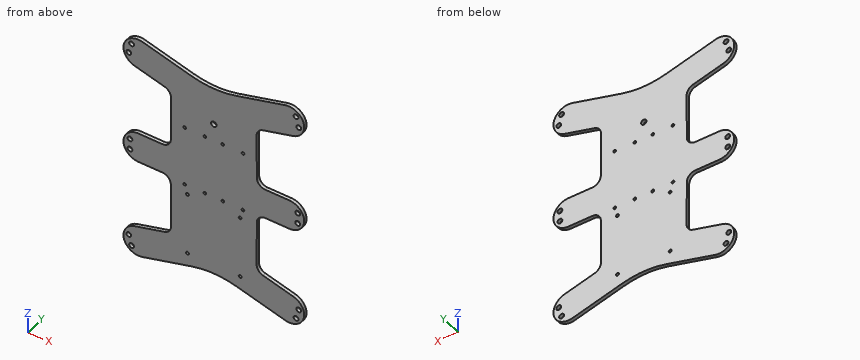
```python
from build123d import *

# Parameters (mm, degrees)
BOSS_EXTRUDE1_DEPTH = 3.175
FILLET1_R           = 80
FILLET2_R           = 8
SKETCH2_R           = 1.35
CUT_EXTRUDE1_DEPTH  = 136.741386774
SKETCH3_R           = 1.25
CUT_EXTRUDE2_DEPTH  = 136.741386774
SKETCH5_R           = 2.55
CUT_EXTRUDE3_DEPTH  = 136.741386774
SKETCH7_R           = 2.25
CUT_EXTRUDE4_DEPTH  = 10


with BuildPart() as part:
    # Sketch1 → Boss-Extrude1 (new body)
    with BuildSketch(Plane(origin=(0, 0, 0), x_dir=(1, 0, 0), z_dir=(0, 1, 0))):
        with BuildLine():
            Line((-70, 14), (-40, 14))
            Line((-40, 14), (-39.816062711, 70))
            Line((-39.816062711, 70), (-73.623466631, 79.058666579))
            ThreePointArc((-73.623466631, 79.058666579), (-83.522961568, 96.205094778), (-66.376533369, 106.104589715))
            Line((-66.376533369, 106.104589715), (0, 88.319051202))
            Line((0, 88.319051202), (66.376533369, 106.104589715))
            ThreePointArc((66.376533369, 106.104589715), (83.522961568, 96.205094778), (73.623466631, 79.058666579))
            Line((73.623466631, 79.058666579), (39.816062711, 70))
            Line((39.816062711, 70), (40, 14))
            Line((40, 14), (70, 14))
            ThreePointArc((70, 14), (84, 0), (70, -14))
            Line((70, -14), (40, -14))
            Line((40, -14), (39.816062711, -70))
            Line((39.816062711, -70), (73.623466631, -79.058666579))
            ThreePointArc((73.623466631, -79.058666579), (83.522961568, -96.205094778), (66.376533369, -106.104589715))
            Line((66.376533369, -106.104589715), (0, -88.319051202))
            Line((0, -88.319051202), (-66.376533369, -106.104589715))
            ThreePointArc((-66.376533369, -106.104589715), (-83.522961568, -96.205094778), (-73.623466631, -79.058666579))
            Line((-73.623466631, -79.058666579), (-39.816062711, -70))
            Line((-39.816062711, -70), (-40, -14))
            Line((-40, -14), (-70, -14))
            ThreePointArc((-70, -14), (-84, 0), (-70, 14))
        make_face()
    extrude(amount=BOSS_EXTRUDE1_DEPTH)

    # Fillet1
    fillet1_edges = [part.edges().sort_by_distance(p)[0] for p in [
        (0, 1.5875, -88.319051202),
        (0, 1.5875, 88.319051202),
    ]]
    fillet(fillet1_edges, radius=FILLET1_R)

    # Fillet2
    fillet2_edges = [part.edges().sort_by_distance(p)[0] for p in [
        (-40, 1.5875, -14),
        (-39.816062711, 1.5875, -70),
        (39.816062711, 1.5875, -70),
        (40, 1.5875, -14),
        (40, 1.5875, 14),
        (39.816062711, 1.5875, 70),
        (-39.816062711, 1.5875, 70),
        (-40, 1.5875, 14),
    ]]
    fillet(fillet2_edges, radius=FILLET2_R)

    # Sketch2 → Cut-Extrude1 (cut, through all)
    with BuildSketch(Plane(origin=(0, 3.175, 0), x_dir=(1, 0, 0), z_dir=(0, 1, 0))):
        with Locations(Location((-24.5, 24.641145635, 0), (0, 0, 270))):
            Circle(SKETCH2_R)
        with Locations(Location((24.5, 24.641145635, 0), (0, 0, 270))):
            Circle(SKETCH2_R)
        with Locations(Location((24.5, 82.641145635, 0), (0, 0, 270))):
            Circle(SKETCH2_R)
        with Locations(Location((-24.5, 82.641145635, 0), (0, 0, 270))):
            Circle(SKETCH2_R)
    extrude(amount=-CUT_EXTRUDE1_DEPTH, mode=Mode.SUBTRACT)

    # Sketch3 → Cut-Extrude2 (cut, through all)
    with BuildSketch(Plane(origin=(0, 3.175, 0), x_dir=(1, 0, 0), z_dir=(0, 1, 0))):
        with Locations(Location((-8.3, -40.058854365, 0), (0, 0, 270))):
            Circle(SKETCH3_R)
        with Locations(Location((-27.1, -40.058854365, 0), (0, 0, 270))):
            Circle(SKETCH3_R)
        with Locations(Location((-27.1, 15.841145635, 0), (0, 0, 270))):
            Circle(SKETCH3_R)
        with Locations(Location((-8.3, 15.841145635, 0), (0, 0, 270))):
            Circle(SKETCH3_R)
        with Locations(Location((8.3, 15.841145635, 0), (0, 0, 270))):
            Circle(SKETCH3_R)
        with Locations(Location((27.1, 15.841145635, 0), (0, 0, 270))):
            Circle(SKETCH3_R)
        with Locations(Location((8.3, -40.058854365, 0), (0, 0, 270))):
            Circle(SKETCH3_R)
        with Locations(Location((27.1, -40.058854365, 0), (0, 0, 270))):
            Circle(SKETCH3_R)
    extrude(amount=-CUT_EXTRUDE2_DEPTH, mode=Mode.SUBTRACT)

    # Sketch5 → Cut-Extrude3 (cut, through all)
    with BuildSketch(Plane(origin=(0, 3.175, 0), x_dir=(1, 0, 0), z_dir=(0, 1, 0))):
        with Locations(Location((0, -56.018854365, 0), (0, 0, 270))):
            Circle(SKETCH5_R)
    extrude(amount=-CUT_EXTRUDE3_DEPTH, mode=Mode.SUBTRACT)

    # Sketch7 → Cut-Extrude4 (cut)
    with BuildSketch(Plane(origin=(0, 3.175, 0), x_dir=(1, 0, 0), z_dir=(0, 1, 0))):
        with Locations(Location((-76.433311385, -99.481809639, 0), (0, 0, 270))):
            Circle(SKETCH7_R)
        with Locations(Location((-79.021501836, -89.822551376, 0), (0, 0, 270))):
            Circle(SKETCH7_R)
        with Locations(Location((-78, -5, 0), (0, 0, 270))):
            Circle(SKETCH7_R)
        with Locations(Location((-78, 5, 0), (0, 0, 270))):
            Circle(SKETCH7_R)
        with Locations(Location((-79.021501836, 89.822551376, 0), (0, 0, 270))):
            Circle(SKETCH7_R)
        with Locations(Location((-76.433311385, 99.481809639, 0), (0, 0, 270))):
            Circle(SKETCH7_R)
        with Locations(Location((79.021501836, 89.822551376, 0), (0, 0, 270))):
            Circle(SKETCH7_R)
        with Locations(Location((76.433311385, 99.481809639, 0), (0, 0, 270))):
            Circle(SKETCH7_R)
        with Locations(Location((78, -5, 0), (0, 0, 270))):
            Circle(SKETCH7_R)
        with Locations(Location((78, 5, 0), (0, 0, 270))):
            Circle(SKETCH7_R)
        with Locations(Location((79.021501836, -89.822551376, 0), (0, 0, 270))):
            Circle(SKETCH7_R)
        with Locations(Location((76.433311385, -99.481809639, 0), (0, 0, 270))):
            Circle(SKETCH7_R)
    extrude(amount=-CUT_EXTRUDE4_DEPTH, mode=Mode.SUBTRACT)


solid = part.part
```
The listing builds one solid part. Answer for the finished solid, in the listing's coordinates (mm). Give positions to 0.01 mm unless a question says otherwise; leave off trailing zeros. Write each loop counter-clockwise with the first axis right and the second up, starting at its lowest first coordinate (ties: lowest second). Pieces come first, ordered by that corner, then holes. Notation, with made-up numbers: (77, 71.5) - (117, 71.5) arc R16 cw to (117, 90.5) - close; hole circle Ø1 at (28.5, 45). An arc over 180 degrees is marked (long way). Use one line per item in the form item = value. Start each with the question number.
1) Find section D-D on y = 1.95. Count the separate pieces of the cut face and the enclosed holes in it, plus the area to 3 significant figures.
2) Find section B-B on x = -43.5. Determine the outline of the cut face in (y, z) (3 decimals).
3) Flat-ended cylindrical pins translate along their axes: pin 1 Ø1 at (x, y) = (63.5, 1.5) entering from -Z; pin 2 Ø6 at (x, z) = (76.43, 99.48) entering from -Y; pin 3 Ø1.5 at (x, z) = (8.3, -15.84) entering from +Y; pin 4 Ø1 at (x, y) = (16.5, 3) entering from -Z. Find the tip coordinate at first contact, or state that the pin passes through.
4) Find section C-C on z = -5. Determine the outline of the cut face in (x, y) (3 decimals).
5) Consider line 1 along Z through (x, y) = (-70.5, 1.6); line 2 along Z through (x, y) = (73.5, 2.95); line 3 along X through (y, z) = (2.7, 89.5). Determine where each line is inside the solid, lowest interval first. Write a range as from..to.
6) Find section A-A on x = 0. Determine the outline of the cut face in (y, z) (3 decimals).
Geometry results:
q1.separate_pieces = 1
q1.enclosed_holes = 25
q1.area = 21,900 mm2
q2.outline = (0, -99.975) - (3.175, -99.975) - (3.175, -70.59) - (0, -70.59) - close; (0, -15.368) - (3.175, -15.368) - (3.175, 15.368) - (0, 15.368) - close; (0, 70.59) - (3.175, 70.59) - (3.175, 99.975) - (0, 99.975) - close
q3.pin_1 = -105.47
q3.pin_2 = 0
q3.pin_3 = through
q3.pin_4 = -92.97
q4.outline = (-83.077, 0) - (-80.25, 0) - (-80.25, 3.175) - (-83.077, 3.175) - close; (-75.75, 0) - (75.75, 0) - (75.75, 3.175) - (-75.75, 3.175) - close; (80.25, 0) - (83.077, 0) - (83.077, 3.175) - (80.25, 3.175) - close
q5.line_1 = -106.57..-78.22, -13.99..13.99, 78.22..106.57
q5.line_2 = -106.14..-79.03, -13.56..13.56, 79.03..106.14
q5.line_3 = -83.66..-81.25, -76.79..76.79, 81.25..83.66
q6.outline = (0, -91.141) - (3.175, -91.141) - (3.175, 53.469) - (0, 53.469) - close; (0, 58.569) - (3.175, 58.569) - (3.175, 91.141) - (0, 91.141) - close
